Verification items for the finished model (mm, model axes). A direction names the side the tool comes from. Round coordinates to 2 decimals unless told otherwise and drop trailing zeros. Write each loop counter-clockwise with the first axis right and the second up, starting at its lowest first coordinate (ties: lowest second). Pieces come first, ordered by that corner, then holes.
from build123d import *

# Parameters (mm, degrees)
SKETCH1_R           = 11
BOSS_EXTRUDE1_DEPTH = 10
SKETCH2_W           = 3
SKETCH2_H           = 5


with BuildPart() as part:
    # Sketch1 → Boss-Extrude1 (new body)
    with BuildSketch(Plane.XY):
        Circle(SKETCH1_R)
        with BuildLine():
            ThreePointArc((1.8, -2.4), (0, 3), (-1.8, -2.4))
            Line((-1.8, -2.4), (1.8, -2.4))
        make_face(mode=Mode.SUBTRACT)
    extrude(amount=BOSS_EXTRUDE1_DEPTH)

    # Sketch2 → Cut-Revolve1 (revolve, cut)
    with BuildSketch(Plane(origin=(0, 0, 0), x_dir=(1, 0, 0), z_dir=(0, 1, 0))):
        with Locations((-9.5, -5)):
            Rectangle(SKETCH2_W, SKETCH2_H)
    revolve(axis=Axis((0, 0, 0), (0, 0, 1)), mode=Mode.SUBTRACT)


solid = part.part
Q1. Sectioned sample at A-A (y = 0). Enter the section's corners in (x, z), plus the area to 3 significant figures.
Recorded:
outline: (-11, 0) - (-3, 0) - (-3, 10) - (-11, 10) - (-11, 7.5) - (-8, 7.5) - (-8, 2.5) - (-11, 2.5) - close; (3, 0) - (11, 0) - (11, 2.5) - (8, 2.5) - (8, 7.5) - (11, 7.5) - (11, 10) - (3, 10) - close
area: 130 mm2
Q2. Tool access check on faces 4 (the flat face through (2, 8, 7.5)), 5 (the cylindrical face through (-2.38, -10.74, 8.73)). Record the directions out of +Z, -Z, +X, -X, +Y, -Y that give a thin tool (end or side, any length) a straight path to the whole face; none if there is none.
Recorded:
face 4: none
face 5: +Z, -Z
Q3. Sectioned sample at B-B (x = 0). Enter the section's corners in (y, z), plus the area to 3 significant figures.
Recorded:
outline: (-11, 0) - (-2.4, 0) - (-2.4, 10) - (-11, 10) - (-11, 7.5) - (-8, 7.5) - (-8, 2.5) - (-11, 2.5) - close; (3, 0) - (11, 0) - (11, 2.5) - (8, 2.5) - (8, 7.5) - (11, 7.5) - (11, 10) - (3, 10) - close
area: 136 mm2
Q4. Material ranges on line 1 along Z through (x, y) = (0.25, 10); line 2 along Y through (x, z) = (0, 6); line 3 along X through (y, z) = (0, 4.5), recorded low to high.
Recorded:
line 1: z = 0 to 2.5, 7.5 to 10
line 2: y = -8 to -2.4, 3 to 8
line 3: x = -8 to -3, 3 to 8
Q5. Sectioned sample at C-C (z = 1.5). Enter the section's corners in (x, y).
Recorded:
outline: circle Ø22 at (0, 0); hole (-1.8, -2.4) - (1.8, -2.4) arc R3 ccw (long way) to start
Q6. Depth check by flat-ended pin: P1, Ø1, axis at x = 2, z = 4, coming from the -Y side; P2, Ø2, axis at x = 5.5, z = 8.5, coming from the +Y side; P3, Ø1.5, axis at x = -8, z = 3.5, coming from the -Y side. Enter the tip coordinate at first touch or a pass-through.
Recorded:
P1: stops at y = -7.86
P2: stops at y = 10.04
P3: stops at y = -3.38
Q7. Release check for a two-part mould opening along Z. For faces 1 (the flat face through (2.3, -2.3, 10)), 2 (the cylindrical face through (1.73, 7.81, 4.96)), 3 (the flat face through (0, -2.4, 5)) record: released by +Z, released by -Z, zero draft, split by the parting line, or undercut.
Recorded:
face 1: released by +Z
face 2: undercut
face 3: zero draft
Q8. Sectioned sample at D-D (x = 5.75). Enter the section's corners in (y, z), plus the area to 3 significant figures.
Recorded:
outline: (-9.38, 0) - (9.38, 0) - (9.38, 2.5) - (5.56, 2.5) - (5.56, 7.5) - (9.38, 7.5) - (9.38, 10) - (-9.38, 10) - (-9.38, 7.5) - (-5.56, 7.5) - (-5.56, 2.5) - (-9.38, 2.5) - close
area: 149 mm2
